from build123d import *

# Parameters (mm, degrees)
SKETCH1_R           = 3.5
BOSS_EXTRUDE1_DEPTH = 3.175


with BuildPart() as part:
    # Sketch1 → Boss-Extrude1 (new body)
    with BuildSketch(Plane(origin=(0, 0, 0), x_dir=(1, 0, 0), z_dir=(0, 1, 0))):
        with BuildLine():
            Line((-7.559940761, 17.117095983), (-6.363973726, 22.870814531))
            ThreePointArc((-6.363973726, 22.870814531), (0, 28.04799995), (6.363973726, 22.870814531))
            Line((6.363973726, 22.870814531), (7.559940761, 17.117095983))
            ThreePointArc((7.559940761, 17.117095983), (8.292150293, 15.365504727), (9.624553992, 14.013135283))
            ThreePointArc((9.624553992, 14.013135283), (12.02081528, 12.02081528), (14.013135283, 9.624553992))
            ThreePointArc((14.013135283, 9.624553992), (15.365504727, 8.292150293), (17.117095983, 7.559940761))
            Line((17.117095983, 7.559940761), (22.870814531, 6.363973726))
            ThreePointArc((22.870814531, 6.363973726), (28.04799995, 0), (22.870814531, -6.363973726))
            Line((22.870814531, -6.363973726), (17.117095983, -7.559940761))
            ThreePointArc((17.117095983, -7.559940761), (15.365504727, -8.292150293), (14.013135283, -9.624553992))
            ThreePointArc((14.013135283, -9.624553992), (12.02081528, -12.02081528), (9.624553992, -14.013135283))
            ThreePointArc((9.624553992, -14.013135283), (8.292150293, -15.365504727), (7.559940761, -17.117095983))
            Line((7.559940761, -17.117095983), (6.363973726, -22.870814531))
            ThreePointArc((6.363973726, -22.870814531), (0, -28.04799995), (-6.363973726, -22.870814531))
            Line((-6.363973726, -22.870814531), (-7.559940761, -17.117095983))
            ThreePointArc((-7.559940761, -17.117095983), (-8.292150293, -15.365504727), (-9.624553992, -14.013135283))
            ThreePointArc((-9.624553992, -14.013135283), (-12.02081528, -12.02081528), (-14.013135283, -9.624553992))
            ThreePointArc((-14.013135283, -9.624553992), (-15.365504727, -8.292150293), (-17.117095983, -7.559940761))
            Line((-17.117095983, -7.559940761), (-22.870814531, -6.363973726))
            ThreePointArc((-22.870814531, -6.363973726), (-28.04799995, 0), (-22.870814531, 6.363973726))
            Line((-22.870814531, 6.363973726), (-17.117095983, 7.559940761))
            ThreePointArc((-17.117095983, 7.559940761), (-15.365504727, 8.292150293), (-14.013135283, 9.624553992))
            ThreePointArc((-14.013135283, 9.624553992), (-12.02081528, 12.02081528), (-9.624553992, 14.013135283))
            ThreePointArc((-9.624553992, 14.013135283), (-8.292150293, 15.365504727), (-7.559940761, 17.117095983))
        make_face()
        with Locations((0, 21.54799995)):
            Circle(SKETCH1_R, mode=Mode.SUBTRACT)
        with Locations((21.54799995, 0)):
            Circle(SKETCH1_R, mode=Mode.SUBTRACT)
        with Locations((0, -21.54799995)):
            Circle(SKETCH1_R, mode=Mode.SUBTRACT)
        with Locations((-21.54799995, 0)):
            Circle(SKETCH1_R, mode=Mode.SUBTRACT)
    extrude(amount=BOSS_EXTRUDE1_DEPTH)


solid = part.part
CAD build for the part. Positions are in the model's coordinates, mm. Give positions to 0.01 mm unless a question says otherwise; leave off trailing zeros. Loops run counter-clockwise (first coordinate to the right, second up) from the corner with the lowest first, then second, coordinate; pieces in that order, holes last. Notation, with made-up numbers: M -35,-40 L -23,-40 A20 ccw -23,-11 Z; hole C 35,53.25 d2. An arc over 180 degrees is marked long. Answer in a Markdown table with one row per item. Add a question column.
Item 1: Band-saw the part on A-A on z = 0. Give the cut face in (x, y) (3 decimals), then the cut area to 3 significant figures.
Item 2: Drop flat-ended pins along their axis: P1, Ø1, axis at x = 21.5, y = 2.5, coming from the -Z side; P2, Ø1, axis at y = 2, z = 15.5, coming from the +X side. Give the stop position or say it passes through.
Item 3: Probe probe 1 along X at (y, z) = (1.9, -2.5); probe 2 along X at (y, z) = (1.3, -24.5); probe 3 along X at (y, z) = (1.2, -22). List the from-to ranges inside material, lowest first.
Item 4: Band-saw the part on B-B on x = 0. Give the cut face in (y, z) (3 decimals), then the cut area to 3 significant figures.
Item 5: Band-saw the part on D-D on z = 19.5. Give the cut face in (x, y) (3 decimals), then the cut area to 3 significant figures.
Item 6: Band-saw the part on C-C on y = 1.5. Give the cut face in (x, z), then the cut area to 3 significant figures.
Reply:
| question | item | result |
|---|---|---|
| 1 | outline | M -28.048,0 L -25.048,0 L -25.048,3.175 L -28.048,3.175 Z; M -18.048,0 L 18.048,0 L 18.048,3.175 L -18.048,3.175 Z; M 25.048,0 L 28.048,0 L 28.048,3.175 L 25.048,3.175 Z |
| 1 | area | 134 mm^2 |
| 2 | P1 | stops at z = -6.75 |
| 2 | P2 | stops at x = 8.56 |
| 3 | probe 1 | x = -27.55 to -24, -19.1 to 19.1, 24 to 27.55 |
| 3 | probe 2 | x = -5.79 to -1.88, 1.88 to 5.79 |
| 3 | probe 3 | x = -6.54 to -3.47, 3.47 to 6.54 |
| 4 | outline | M 0,-28.048 L 3.175,-28.048 L 3.175,-25.048 L 0,-25.048 Z; M 0,-18.048 L 3.175,-18.048 L 3.175,18.048 L 0,18.048 Z; M 0,25.048 L 3.175,25.048 L 3.175,28.048 L 0,28.048 Z |
| 4 | area | 134 mm^2 |
| 5 | outline | M -7.065,0 L -2.838,0 L -2.838,3.175 L -7.065,3.175 Z; M 2.838,0 L 7.065,0 L 7.065,3.175 L 2.838,3.175 Z |
| 5 | area | 26.8 mm^2 |
| 6 | outline | M -22.87,-6.36 L -17.12,-7.56 A5 cw -14.01,-9.62 A17 ccw -9.62,-14.01 A5 cw -7.56,-17.12 L -6.36,-22.87 A6.5 ccw 6.36,-22.87 L 7.56,-17.12 A5 cw 9.62,-14.01 A17 ccw 14.01,-9.62 A5 cw 17.12,-7.56 L 22.87,-6.36 A6.5 ccw 22.87,6.36 L 17.12,7.56 A5 cw 14.01,9.62 A17 ccw 9.62,14.01 A5 cw 7.56,17.12 L 6.36,22.87 A6.5 ccw -6.36,22.87 L -7.56,17.12 A5 cw -9.62,14.01 A17 ccw -14.01,9.62 A5 cw -17.12,7.56 L -22.87,6.36 A6.5 ccw Z; hole C -21.55,0 d7; hole C 0,-21.55 d7; hole C 0,21.55 d7; hole C 21.55,0 d7 |
| 6 | area | 1,320 mm^2 |
